Design review of the part built by this model. Coordinates are the model's own, in mm. Face numbers are marked on the shaded views. A direction names the side the tool comes from. Coordinates: 2 decimals unless noted, no trailing zeros. Loops run counter-clockwise (first coordinate to the right, second up) from the corner with the lowest first, then second, coordinate; pieces in that order, holes last. Notation, with made-up numbers: M -8.5,71.25 L 31.5,71.25 A19 ccw 31.5,75.25 Z; hole C 20,39.25 d11. An arc over 180 degrees is marked long. Answer as a JSON object with one key per item and string values. Group by question number.
1. Machinability: for the marked faces 4 and 5, which of the approach directions +Z, -Z, +X, -X, +Y, -Y give a long, thin tool a straight path to every point of the face, cutting with its end or side? Answer none if there is none.
2. Insertion check: pin 1 (12.5 mm diameter, centred on x = -2, z = 124.5, fed in from -Y); pin 2 (3 mm diameter, centred on x = -48, z = -88.5, fed in from +Y); pin 3 (1 mm diameter, centred on x = 54.5, y = 125, fed in from -Z). Each pin has a flat end and moves straight along its axis. Give the tip position at first contact, or say it passes through.
3. Consider section C-C (y = 25). State the section outline as (x, z) points, then the cut area to 3 significant figures.
4. Consider section B-B (z = -121.5). State the section outline as (x, y) points, then the cut area to 3 significant figures.
5. To check wall thickness, follow probe 1 along X at (y, z) = (129, 0); probe 2 along X at (y, z) = (136, 0); probe 3 along Y at (x, z) = (-59, -85.5). State the ranges of each line that lie inside material, in increasing order.
6. Draft analysis for pull direction Z (two halves, no side actions). For the marked faces 1, 2 and 3, state which applies: +Z half, -Z half, draft (parallel to the pull), parting line (faces both ways), or undercut.
7. Consider section A-A (y = 50). State the section outline as (x, z) points (3 decimals).
from build123d import *

# Parameters (mm, degrees)
FILLET1_R                    = 37.5
FILLET6_R                    = 37.5
FILLET8_R                    = 22.5
SKETCH4_R                    = 9.749999999999996
BOSS_EXTRUDE2_DEPTH          = 30
CHAMFER1_SIZE                = 2
CIRPATTERN4_COUNT            = 6
CHAMFER1_OF_CIRPATTERN4_SIZE = 2


with BuildPart() as part:
    # Sketch1 → Revolve1 (revolve)
    with BuildSketch(Plane.XY, mode=Mode.PRIVATE) as revolve1_sk:
        Polygon((0, 0), (-45, 0), (-45, 44.99999999999999), (-75.00000000000001, 44.999999999999986), (-75.00000000000001, 59.07407407407406), (-135, 59.074074074074055), (-135, 89.07407407407406), (-60, 89.07407407407405), (-60, 164.07407407407405), (-45.00000000000001, 164.07407407407405), (-45, 119.07407407407403), (0, 119.07407407407403), align=None)
    revolve(revolve1_sk.sketch.rotate(Axis((0, 119.07407407407403, 0), (0, -1, 0)), 270), axis=Axis((0, 119.07407407407403, 0), (0, -1, 0)))

    # Fillet1
    # the kernel refuses this fillet: 37.5 mm, written as the material it adds along each edge
    with BuildSketch(Plane(origin=(0, 89.07407407407405, 0), x_dir=(2.2e-16, 0, 1), z_dir=(1, 0, -2.2e-16))) as fillet1_piece_1:
        with BuildLine():
            CenterArc((60 + FILLET1_R, -FILLET1_R), FILLET1_R, 90, 89.99999999999997)
            Line((60, -FILLET1_R), (60, 0))
            Line((60, 0), (60 + FILLET1_R, -1.421e-14))
        make_face()
    revolve(axis=Axis((0, 89.07407407407405, 0), (0, -1, 0)))
    # the kernel refuses this fillet: 37.5 mm, written as the material it takes off along each edge
    with BuildSketch(Plane(origin=(0, 164.07407407407405, 0), x_dir=(2.2e-16, 0, 1), z_dir=(1, 0, -2.2e-16))) as fillet1_2_piece_1:
        with BuildLine():
            CenterArc((22.5, 30), FILLET1_R, 306.86989764584405, 53.13010235415595)
            Line((45.00000000000001, 0), (60, 0))
            Line((60, 0), (60, 30))
        make_face()
    revolve(axis=Axis((0, 164.07407407407405, 0), (0, -1, 0)), mode=Mode.SUBTRACT)

    # Fillet6
    # the kernel refuses this fillet: 37.5 mm, written as the material it adds along each edge
    with BuildSketch(Plane(origin=(0, 44.999999999999986, 0), x_dir=(2.2e-16, 0, 1), z_dir=(1, 0, -2.2e-16))) as fillet6_piece_1:
        with BuildLine():
            CenterArc((82.5, 36.742346141747674), FILLET6_R, 180, 78.4630409671845)
            Line((45, 36.742346141747674), (44.25, 36.742346141747674))
            Line((44.25, 36.742346141747674), (44.25, 0))
            Line((44.25, 0), (45, -0.75))
            ThreePointArc((45, -0.75), (60.00000000000001, -0.75), (74.85000000000001, -0.7348469228349543))
            Line((74.85000000000001, -0.7348469228349543), (75.00000000000001, 0))
        make_face()
    revolve(axis=Axis((0, 44.999999999999986, 0), (0, -1, 0)))

    # Fillet8
    fillet8_edges = [part.edges().sort_by_distance(p)[0] for p in [
        (-1.55e-14, 0, -45),
    ]]
    fillet(fillet8_edges, radius=FILLET8_R)

    # Sketch4 → Boss-Extrude2 (add)
    with BuildSketch(Plane.XZ.offset(-59.074074074074055)):
        with Locations(Location((0, 121.5, 0), (0, 0, 270))):
            Circle(SKETCH4_R)
    boss_extrude2 = extrude(amount=BOSS_EXTRUDE2_DEPTH)

    # Chamfer1
    chamfer1_edges = [part.edges().sort_by_distance(p)[0] for p in [
        (2.99e-15, 29.074074074074055, 131.25),
    ]]
    chamfer(chamfer1_edges, length=CHAMFER1_SIZE)

    # CirPattern4: Boss-Extrude2 ×6 about axis
    cirpattern4_axis = Axis((1.4387e-13, 0, -3.74e-15), (0, 1, 0))
    for i in range(1, CIRPATTERN4_COUNT):
        add(boss_extrude2.rotate(cirpattern4_axis, i * 360 / CIRPATTERN4_COUNT))

    # Chamfer1 of CirPattern4
    chamfer1_of_cirpattern4_edges = [part.edges().sort_by_distance(p)[0] for p in [
        (113.66583424670763, 29.074074074074055, 65.62500000000014),
        (113.66583424670779, 29.074074074074055, -65.62499999999986),
        (3.0083e-13, 29.074074074074055, -131.25),
        (-113.66583424670732, 29.074074074074055, -65.62500000000018),
        (-113.66583424670749, 29.074074074074055, 65.62499999999989),
    ]]
    chamfer(chamfer1_of_cirpattern4_edges, length=CHAMFER1_OF_CIRPATTERN4_SIZE)


solid = part.part
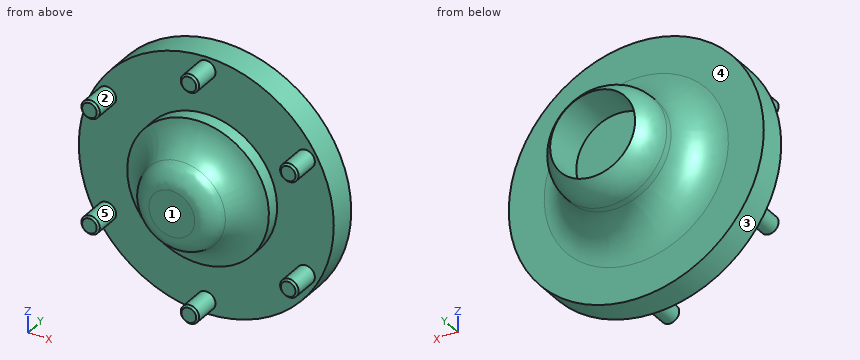
Findings below:
{
 "1": {"face 4": "+Y", "face 5": "-Y"},
 "2": {"pin 1": "stops at y = 29.07", "pin 2": "stops at y = 89.07", "pin 3": "stops at z = -26.23"},
 "3": {"outline": "C 0,0 d97.89", "area": "7,530 mm^2"},
 "4": {"outline": "M -58.85,59.07 L -9.75,59.07 L -9.75,31.07 L -7.75,29.07 L 7.75,29.07 L 9.75,31.07 L 9.75,59.07 L 58.85,59.07 L 58.85,89.07 L -58.85,89.07 Z", "area": "4,110 mm^2"},
 "5": {"probe 1": "x = -60 to -45, 45 to 60", "probe 2": "x = -59.95 to -45, 45 to 59.95", "probe 3": "y = 59.07 to 89.07"},
 "6": {"face 1": "draft", "face 2": "undercut", "face 3": "parting line"},
 "7": {"outline": "C -105.222,-60.75 d19.5; C -105.222,60.75 d19.5; C 0,0 d150; C 0,-121.5 d19.5; C 0,121.5 d19.5; C 105.222,-60.75 d19.5; C 105.222,60.75 d19.5"}
}
